Here's how the part is built. I have some questions about the finished solid (model axes, mm). Round coordinates to 2 decimals unless told otherwise and drop trailing zeros. Write each loop counter-clockwise with the first axis right and the second up, starting at its lowest first coordinate (ties: lowest second). Pieces come first, ordered by that corner, then holes. Notation, with made-up numbers: M 47.5,-2 L 54.5,-2 A13 cw 54.5,11 Z; hole C -14.5,-38 d6. An arc over 180 degrees is marked long. Use a Markdown table: item, result. Add a question column.
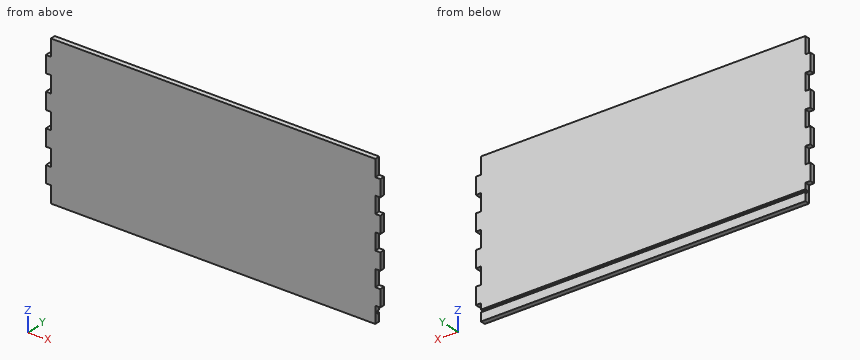
```python
from build123d import *

# Parameters (mm, degrees)
F0_W     = 400
F0_H     = 6
F1_DEPTH = 180
F2_W     = 3
F2_H     = 3
F3_DEPTH = 400.001
F4_W     = 6
F4_H     = 20
F5_DEPTH = 6.001


with BuildPart() as f1:
    # F0 (on Top) → F1 (new body)
    with BuildSketch(Plane.XY):
        Rectangle(F0_W, F0_H)
    extrude(amount=F1_DEPTH)

    # F2 (on face) → F3 (cut, through all)
    with BuildSketch(Plane.YZ.offset(200)):
        with Locations((1.5, 11.5)):
            Rectangle(F2_W, F2_H)
    extrude(amount=-F3_DEPTH, mode=Mode.SUBTRACT)

    # F4 (on face) → F5 (cut, through all)
    with BuildSketch(Plane.XZ.offset(3)):
        with Locations((-197, 170)):
            Rectangle(F4_W, F4_H)
        with Locations((-197, 130)):
            Rectangle(F4_W, F4_H)
        with Locations((-197, 90)):
            Rectangle(F4_W, F4_H)
        with Locations((-197, 50)):
            Rectangle(F4_W, F4_H)
        with Locations((-197, 10)):
            Rectangle(F4_W, F4_H)
        with Locations((197, 10)):
            Rectangle(F4_W, F4_H)
        with Locations((197, 50)):
            Rectangle(F4_W, F4_H)
        with Locations((197, 90)):
            Rectangle(F4_W, F4_H)
        with Locations((197, 130)):
            Rectangle(F4_W, F4_H)
        with Locations((197, 170)):
            Rectangle(F4_W, F4_H)
    extrude(amount=-F5_DEPTH, mode=Mode.SUBTRACT)


solid = f1.part
```
Item 1: I need wall thicknesses on probe 1 along Z at (x, y) = (52.5, 1.15); probe 2 along Y at (x, z) = (-184, 11); probe 3 along X at (y, z) = (-2.05, 44). Which ranges of each line are inside material? Lowest first, please. Write a range as from..to.
Item 2: Imagine slicing it at A-A on z = 131.5. List the corners of the cut face in (x, y) for me, plus the area to 3 significant figures.
Item 3: For pin 1 Ø1.8 at (x, y) = (-198.5, -1) entering from -Z; pin 2 Ø1.8 at (x, y) = (-196.5, 1) entering from +Z; pin 3 Ø1.8 at (y, z) = (-0.5, 167.5) entering from +X, each with a flat end and sliding along its axis, tell me the tip position at first contact or that it passes through.
The answers:
| question | item | result |
|---|---|---|
| 1 | probe 1 | 0..10, 13..180 |
| 1 | probe 2 | -3..0 |
| 1 | probe 3 | -194..194 |
| 2 | outline | M -194,-3 L 194,-3 L 194,3 L -194,3 Z |
| 2 | area | 2,330 mm² |
| 3 | pin 1 | z = 20 |
| 3 | pin 2 | z = 160 |
| 3 | pin 3 | x = 194 |
